Part print with two shaded views. Sizes in mm from the minimum x, y, z corner. A direction names the side the tool comes from. Round coordinates to 2 decimals unless told otherwise and drop trailing zeros. Write each loop counter-clockwise with the first axis right and the second up, starting at its lowest first coordinate (ties: lowest second). Pieces come first, ordered by that corner, then holes. Notation, with made-up numbers: (76.25, 49.5) -> (117.25, 49.5) arc R31 cw to (117.25, 84.5) -> close; hole circle Ø5 at (29.25, 41). An arc over 180 degrees is marked (long way). Answer in a Markdown table with one row per item.
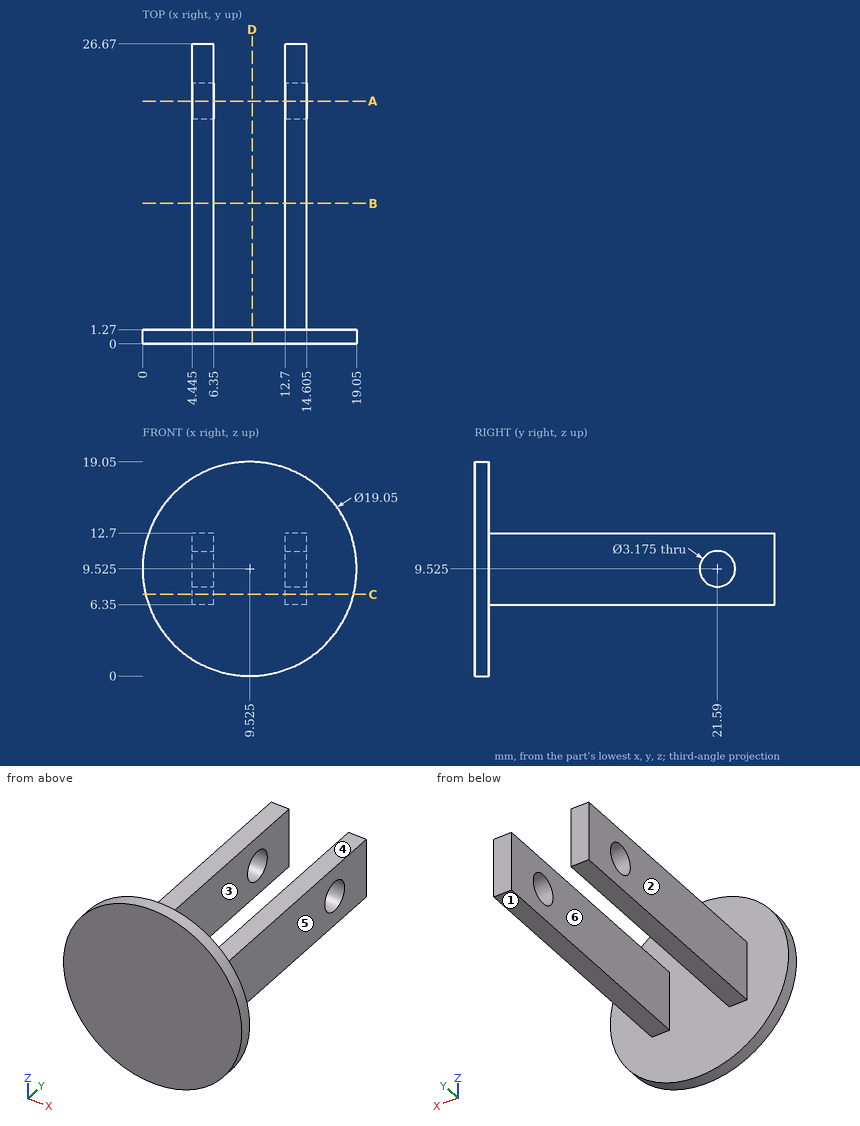
Q1. Saw through at D-D on x = 9.75. Write the cut outline in (y, z), plus the area to 3 significant figures.
A:
| item | result |
|---|---|
| outline | (0, 0) -> (1.27, 0) -> (1.27, 19.05) -> (0, 19.05) -> close |
| area | 24.2 mm² |
Q2. Two-plate mould, pull along X, no slides. Class the marked faces 4, 5 and 6: released by +X, released by -X, zero draft, split by the parting line, or undercut.
A:
| item | result |
|---|---|
| face 4 | zero draft |
| face 5 | released by +X |
| face 6 | undercut |
Q3. Saw through at B-B on y = 12.5. Write the cut outline in (x, z) (3 decimals).
A:
| item | result |
|---|---|
| outline | (4.445, 6.35) -> (6.35, 6.35) -> (6.35, 12.7) -> (4.445, 12.7) -> close; (12.7, 6.35) -> (14.605, 6.35) -> (14.605, 12.7) -> (12.7, 12.7) -> close |
Q4. Saw through at C-C on z = 7.25. Write the cut outline in (x, y) (3 decimals), plus the area to 3 significant figures.
A:
| item | result |
|---|---|
| outline | (0.276, 0) -> (18.774, 0) -> (18.774, 1.27) -> (14.605, 1.27) -> (14.605, 26.67) -> (12.7, 26.67) -> (12.7, 1.27) -> (6.35, 1.27) -> (6.35, 26.67) -> (4.445, 26.67) -> (4.445, 1.27) -> (0.276, 1.27) -> close |
| area | 120 mm² |
Q5. Which spindle directions (+Z, -Z, +X, -X, +Y, -Y) get a long thin tool onto all of the face, cutting with end or side? Do the marked faces 1, 2 and 3. Say none if no direction does.
A:
| item | result |
|---|---|
| face 1 | -Z, +X, -X, +Y |
| face 2 | +Z, -Z, -X, +Y |
| face 3 | +Z, -Z, +Y |
Q6. Wall check: line 1 (Z direction, x = 13.25, y = 21.59); line 2 (X direction, y = 24.75, z = 9.5) (3 decimals); line 3 (Y direction, x = 4.25, z = 3.5). Give the ranges that are in metal, low to high. Write a range as [from, to].
A:
| item | result |
|---|---|
| line 1 | [6.35, 7.94], [11.11, 12.7] |
| line 2 | [4.445, 6.35], [12.7, 14.605] |
| line 3 | [0, 1.27] |
Q7. Saw through at A-A on y = 21.59. State how many separate pieces and enclosed holes the cut face has, plus the area to 3 significant figures.
A:
| item | result |
|---|---|
| separate pieces | 4 |
| enclosed holes | 0 |
| area | 12.1 mm² |
Q8. Drop flat-ended pins along their axis: P1, Ø3, axis at y = 8, z = 10.5, coming from the +X side (3 decimals); P2, Ø1.5, axis at x = 13, y = 6.5, coming from the +Z side; P3, Ø1.5, axis at x = 13.5, y = 10.5, coming from the -Z side; P4, Ø3, axis at x = 2.5, z = 12, coming from the -Y side. Give the stop position or say it passes through.
A:
| item | result |
|---|---|
| P1 | x = 14.605 |
| P2 | z = 12.7 |
| P3 | z = 6.35 |
| P4 | y = 0 |
